from build123d import *

# Parameters (mm, degrees)
F1_DEPTH = 350
F3_DEPTH = 340.0010036672
F4_R     = 7.5
F5_DEPTH = 5
F6_R     = 7.5
F7_DEPTH = 5


# Not quite as in the source:
# - ends of sketch curves that miss each other by under 0.0002 mm in the source are joined


with BuildPart() as f1:
    # F0 (on Front) → F1 (new body)
    with BuildSketch(Plane.XZ):
        with BuildLine():
            Line((160, -88.7002011906), (-160.0000036672, -88.7002011906))
            ThreePointArc((-160.0000036672, -88.7002011906), (-167.0710714791, -91.6291333788), (-170.0000036672, -98.7002011906))
            Line((-170.0000036672, -98.7002011906), (-170, -148.7002011906))
            Line((-170, -148.7002011906), (-165.0000036672, -148.7002011906))
            Line((-165.0000036672, -148.7002011906), (-165.0000036672, -98.7002011906))
            ThreePointArc((-165.0000036672, -98.7002011906), (-163.5355375731, -95.1646672847), (-160.0000036672, -93.7002011906))
            Line((-160.0000036672, -93.7002011906), (160, -93.7002011906))
            ThreePointArc((160, -93.7002011906), (163.5355339059, -95.1646672847), (165, -98.7002011906))
            Line((165, -98.7002011906), (165, -148.7002011906))
            Line((165, -148.7002011906), (170, -148.7002011906))
            Line((170, -148.7002011906), (170, -98.7002011906))
            ThreePointArc((170, -98.7002011906), (167.0710678119, -91.6291333788), (160, -88.7002011906))
        make_face()
    extrude(amount=F1_DEPTH)

    # F2 (on face) → F3 (cut, through all)
    with BuildSketch(Plane.YZ.offset(170)):
        with BuildLine():
            Line((-66, -148.7002011906), (-50, -148.7002011906))
            Line((-50, -148.7002011906), (-50, -131.7002011906))
            ThreePointArc((-50, -131.7002011906), (-52.3431457505, -126.0433469411), (-58, -123.7002011906))
            ThreePointArc((-58, -123.7002011906), (-63.6568542495, -126.0433469411), (-66, -131.7002011906))
            Line((-66, -131.7002011906), (-66, -148.7002011906))
        make_face()
    extrude(amount=-F3_DEPTH, mode=Mode.SUBTRACT)

    # F4 (on face) → F5 (cut, through all)
    with BuildSketch(Plane.XY.offset(-88.7002011906)):
        with Locations((-100, -300)):
            Circle(F4_R)
        with Locations((100, -300)):
            Circle(F4_R)
    extrude(amount=-F5_DEPTH, mode=Mode.SUBTRACT)

    # F6 (on face) → F7 (join)
    with BuildSketch(Plane.XY.offset(-88.7002011906)):
        with Locations((-75, -200)):
            Circle(F6_R)
        with Locations((-75, -300)):
            Circle(F6_R)
        with Locations((75, -300)):
            Circle(F6_R)
        with Locations((75, -200)):
            Circle(F6_R)
    extrude(amount=F7_DEPTH)


solid = f1.part
Here's how the part is built. I have some questions about the finished solid (model axes, mm). A direction names the side the tool comes from. Give positions to 0.01 mm unless a question says otherwise; leave off trailing zeros. Order: outer loops, then holes, each group sorted by start corner. A loop starts at its lowest first (then second) coordinate and runs counter-clockwise, first axis right, second up. Notation, with made-up numbers: M 4.25,88.5 L 56.25,88.5 A30 cw 56.25,127.5 Z; hole C 71,48.25 d1. An arc over 180 degrees is marked long. Answer as a JSON object with one key per item and string values. Group by question number.
1) On a 3-axis mill with a long thin cutter (end or side, diameter ignored), from which of +Z, -Z, +X, -X, +Y, -Y can I reach the whole of each face in a straight line? I mean faces 5 (the flat face through (-165, -173, -124)), 6 (the flat face through (-1, 0, -92)), 7 (the cylindrical face through (74.024, -192.564, -86.235)). Say none if no direction works.
2) Suppose I cut it at D-D, the plane y = -200. Write out the boundary of the cut face in (x, z), plus the area to 3 significant figures.
3) Please list where these lines run through material, in increasing order: L1, parallel to X at y = -300, z = -90; L2, parallel to Y at x = -100, z = -91; L3, parallel to X at y = -168, z = -128. Write a range as [from, to].
4) We'd pull the mould along Y, two halves only. Please class faces 1 (the cylindrical face through (-75.976, -192.564, -86.235)), 2 (the cylindrical face through (73.37, -307.32, -86.24)), 3 (the flat face through (-2, -173, -93.7)), 4 (the flat face through (-1, -350, -92)): pulls with the +Y half, pulls with the -Y half, needs draft (parallel to the pull), parting line crosses it, or undercut.
5) Suppose I cut it at C-C, the plane x = 75. Write out the boundary of the cut face in (y, z).
6) Suppose I cut it at B-B, the plane x = -100. Write out the boundary of the cut face in (y, z).
7) Suppose I cut it at A-A, the plane y = -300. Write out the boundary of the cut face in (x, z), plus the area to 3 significant figures.
8) I'm going to push flat-ended pins straight in: pin 1 Ø19.5 at (x, y) = (100, -300) entering from +Z; pin 2 Ø13.5 at (x, y) = (-100, -300) entering from +Z; pin 3 Ø5 at (x, y) = (-15.5, -124) entering from -Z; pin 4 Ø1 at (y, z) = (-97, -94.5) entering from +X. Where does each tip first touch, or does it pass through?
Results found:
{
 "1": {"face 5": "-Z, +Y, -Y", "face 6": "+Z, -Z, +X, -X, +Y", "face 7": "+Z"},
 "2": {"outline": "M -170,-148.7 L -165,-148.7 L -165,-98.7 A5 cw -160,-93.7 L 160,-93.7 A5 cw 165,-98.7 L 165,-148.7 L 170,-148.7 L 170,-98.7 A10 ccw 160,-88.7 L 82.5,-88.7 L 82.5,-83.7 L 67.5,-83.7 L 67.5,-88.7 L -67.5,-88.7 L -67.5,-83.7 L -82.5,-83.7 L -82.5,-88.7 L -160,-88.7 A10 ccw -170,-98.7 Z", "area": "2,370 mm²"},
 "3": {"L1": "[-164.93, -107.5], [-92.5, 92.5], [107.5, 164.93]", "L2": "[-350, -307.5], [-292.5, 0]", "L3": "[-170, -165], [165, 170]"},
 "4": {"face 1": "undercut", "face 2": "undercut", "face 3": "needs draft", "face 4": "pulls with the -Y half"},
 "5": {"outline": "M -350,-93.7 L 0,-93.7 L 0,-88.7 L -192.5,-88.7 L -192.5,-83.7 L -207.5,-83.7 L -207.5,-88.7 L -292.5,-88.7 L -292.5,-83.7 L -307.5,-83.7 L -307.5,-88.7 L -350,-88.7 Z"},
 "6": {"outline": "M -350,-93.7 L -307.5,-93.7 L -307.5,-88.7 L -350,-88.7 Z; M -292.5,-93.7 L 0,-93.7 L 0,-88.7 L -292.5,-88.7 Z"},
 "7": {"outline": "M -170,-148.7 L -165,-148.7 L -165,-98.7 A5 cw -160,-93.7 L -107.5,-93.7 L -107.5,-88.7 L -160,-88.7 A10 ccw -170,-98.7 Z; M -92.5,-93.7 L 92.5,-93.7 L 92.5,-88.7 L 82.5,-88.7 L 82.5,-83.7 L 67.5,-83.7 L 67.5,-88.7 L -67.5,-88.7 L -67.5,-83.7 L -82.5,-83.7 L -82.5,-88.7 L -92.5,-88.7 Z; M 107.5,-93.7 L 160,-93.7 A5 cw 165,-98.7 L 165,-148.7 L 170,-148.7 L 170,-98.7 A10 ccw 160,-88.7 L 107.5,-88.7 Z", "area": "2,220 mm²"},
 "8": {"pin 1": "z = -88.7", "pin 2": "through", "pin 3": "z = -93.7", "pin 4": "x = 169.29"}
}
